Read the model definition and answer for the solid it produces. Units are mm, in the model's axes. A direction names the side the tool comes from. Coordinates: 2 decimals unless noted, no trailing zeros. Loops run counter-clockwise (first coordinate to the right, second up) from the corner with the lowest first, then second, coordinate; pieces in that order, holes last.
from build123d import *

# Parameters (mm, degrees)
SCHIZZO1_R               = 5.25
SCHIZZO2_R               = 4
SMUSSO1_SIZE             = 1
SMUSSO1_SIZE2            = 1.172437538
FORO_PER_VITE_M3_1_D     = 5.4
FORO_PER_VITE_M3_1_DEPTH = 7
FORO_PER_VITE_M3_1_TIP   = 1.622323671


with BuildPart() as part:
    # Schizzo1 → Loft1 section 0
    with BuildSketch(Plane(origin=(0, 0, 0), x_dir=(1, 0, 0), z_dir=(0, 1, 0))):
        Circle(SCHIZZO1_R)
    # Schizzo2 → Loft1 section 1
    with BuildSketch(Plane(origin=(0, 9, 0), x_dir=(1, 0, 0), z_dir=(0, 1, 0))):
        Circle(SCHIZZO2_R)
    loft()

    # Smusso1
    smusso1_edges = [part.edges().sort_by_distance(p)[0] for p in [
        (-4, 9, 0),
    ]]
    smusso1_side = [part.faces().sort_by_distance(p)[0] for p in [
        (-4.625, 4.5, 0),
    ]]
    chamfer(smusso1_edges, length=SMUSSO1_SIZE, length2=SMUSSO1_SIZE2, reference=smusso1_side[0])

    # Foro per Vite M3-1
    with Locations(Plane(origin=(0, 0, 0), x_dir=(-1, 0, 0), z_dir=(0, -1, 0))):
        with Locations((0, 0)):
            Hole(FORO_PER_VITE_M3_1_D / 2, depth=FORO_PER_VITE_M3_1_DEPTH)
            with Locations((0, 0, -(FORO_PER_VITE_M3_1_DEPTH + FORO_PER_VITE_M3_1_TIP / 2))):  # 118° drill point
                Cone(0, FORO_PER_VITE_M3_1_D / 2, FORO_PER_VITE_M3_1_TIP, mode=Mode.SUBTRACT)


solid = part.part
Item 1: Determine the mould class of faces 3 (the face through (0.37, 8.34, 0.29)), 4 (the face through (4.35, 4.95, -1.37)), 5 (the face through (0, 9, 0)) for opening direction X: released by +X, released by -X, zero draft, split by the parting line, or undercut.
Numbers:
face 3: undercut
face 4: split by the parting line
face 5: zero draft
Item 2: Find the intervals of material crossed by line 1 along X through (y, z) = (2, -0.5); line 2 along X through (y, z) = (3.5, -1.25); line 3 along Z through (x, y) = (0, 2.25), in increasing order.
Numbers:
line 1: x = -4.95 to -2.65, 2.65 to 4.95
line 2: x = -4.6 to -2.39, 2.39 to 4.6
line 3: z = -4.94 to -2.7, 2.7 to 4.94
Item 3: A cutting plane is placed at A-A on y = 5.75. Determine the outline of the cut face in (x, z).
Numbers:
outline: circle Ø8.9 at (0, 0); hole circle Ø5.4 at (0, 0)
Item 4: Given pin 1 (3 mm diameter, centred on y = 7.5, z = 2.5, fed in from -X); pin 2 (5 mm diameter, centred on y = 3.5, z = -3.5, fed in from -X), each flat-ended and moving along its own axis, determine where each tip first touches the part or whether it passes through.
Numbers:
pin 1: stops at x = -4.14
pin 2: stops at x = -4.75
Item 5: Which of the six approach directions +Z, -Z, +X, -X, +Y, -Y give full straight-line access (tool end or side, diameter ignored) to faces 1 (the face through (2.3, 0, 2.3)), 2 (the face through (-0.585, 3.549, 2.636))?
Numbers:
face 1: +Z, -Z, +X, -X, -Y
face 2: -Y
